Input: part model. Units: mm. Frame: model coordinates. A direction names the side the tool comes from. Coordinates: 2 decimals unless noted, no trailing zeros. Loops run counter-clockwise (first coordinate to the right, second up) from the corner with the lowest first, then second, coordinate; pieces in that order, holes last.
(1) Section C-C, the plane z = -12. Return loops of the section in (x, y).
(2) Section D-D, the plane y = 12. Return loops of the section in (x, z).
(3) Section A-A, the plane z = 0. Return loops of the section in (x, y).
(4) Mould query, pull axis Y, two halves, no side actions, for faces 1 (the face through (-15, -0.762, 1)), 2 (the face through (-20, 20.238, 1)), 3 (the face through (-15.266, 10.836, -49.93)), 4 (the face through (-16, 11, -60)). Classes: released by +Y, released by -Y, zero draft, split by the parting line, or undercut.
(5) Set-up query: faces 5 (the face through (-16, 11, 60)), 6 (the face through (-21, 17.238, 1)). Return all of +Z, -Z, +X, -X, +Y, -Y with unobstructed straight access to the full face (end or side cutting, diameter ignored); none if empty.
(6) Section B-B, the plane z = 50. Return loops of the section in (x, y), then the cut area to 4 significant figures.
(7) Contact query for flat-ended pins moving along their axis: P1, Ø3, axis at y = 9.24, z = -50, coming from the -X side; P2, Ø5, axis at x = -22.78, z = 0, coming from the -Y side. Output: stop coordinate, or through.
(8) Line query: L1, parallel to X at y = 18.05, z = 50; L2, parallel to X at y = 19.4, z = 0; L3, parallel to Y at x = -21.5, z = -43. Output: solid intervals per line, ascending.
```python
from build123d import *

# Parameters (mm, degrees)
EXTRUDE_1_DEPTH     = 60
FILLET_2_R          = 1
FILLET_3_R          = 1
SKETCH_6_R          = 1.6
CUT_EXTRUDE_3_DEPTH = 10
SKETCH_7_R          = 1.6
SKETCH_7_R_2        = 3.879374182
CUT_EXTRUDE_4_DEPTH = 10


with BuildPart() as part:
    # 草图1 → 凸台-拉伸1 (new, symmetric)
    with BuildSketch(Plane.XY):
        Polygon((-13.744850262, -0.762431654), (-13.744850262, 20.237568346), (-24.994850262, 20.237568346), (-24.994850262, 17.237568346), (-16.744850262, 17.237568346), (-16.744850262, -0.762431654), align=None)
    extrude(amount=EXTRUDE_1_DEPTH, both=True)

    # 圆角2
    fillet_2_edges = [part.edges().sort_by_distance(p)[0] for p in [
        (-13.744850262, 20.237568346, 0),
    ]]
    fillet(fillet_2_edges, radius=FILLET_2_R)

    # 圆角3
    fillet_3_edges = [part.edges().sort_by_distance(p)[0] for p in [
        (-16.744850262, 17.237568346, 0),
    ]]
    fillet(fillet_3_edges, radius=FILLET_3_R)

    # 草图6 → 切除-拉伸3 (cut)
    with BuildSketch(Plane.ZY.offset(16.744850262)):
        with Locations(Location((50, 9.237568346, 0), (0, 0, 270))):
            Circle(SKETCH_6_R)
        with Locations(Location((-50, 9.237568346, 0), (0, 0, 270))):
            Circle(SKETCH_6_R)
    extrude(amount=-CUT_EXTRUDE_3_DEPTH, mode=Mode.SUBTRACT)

    # 草图7 → 切除-拉伸4 (cut)
    with BuildSketch(Plane.XZ.offset(-17.237568346)):
        with Locations(Location((-21.994850262, -50, 0), (0, 0, 270))):
            Circle(SKETCH_7_R)
        with Locations(Location((-21.994850262, 50, 0), (0, 0, 270))):
            Circle(SKETCH_7_R)
        with Locations(Location((-22.777733305, 0, 0), (0, 0, 270))):
            Circle(SKETCH_7_R)
        with Locations((-6.137965093, 23.424487804)):
            Circle(SKETCH_7_R_2)
    extrude(amount=-CUT_EXTRUDE_4_DEPTH, mode=Mode.SUBTRACT)


solid = part.part
```
Report:
1. outline: (-24.99, 17.24) - (-17.74, 17.24) arc R1 cw to (-16.74, 16.24) - (-16.74, -0.76) - (-13.74, -0.76) - (-13.74, 19.24) arc R1 ccw to (-14.74, 20.24) - (-24.99, 20.24) - close
2. outline: (-16.74, -60) - (-13.74, -60) - (-13.74, 60) - (-16.74, 60) - close
3. outline: (-24.99, 17.24) - (-24.38, 17.24) - (-24.38, 20.24) - (-24.99, 20.24) - close; (-21.18, 17.24) - (-17.74, 17.24) arc R1 cw to (-16.74, 16.24) - (-16.74, -0.76) - (-13.74, -0.76) - (-13.74, 19.24) arc R1 ccw to (-14.74, 20.24) - (-21.18, 20.24) - close
4. face 1: released by -Y
4. face 2: released by +Y
4. face 3: undercut
4. face 4: zero draft
5. face 5: +Z, +X, -X, +Y, -Y
5. face 6: +Z, -Z, -X, -Y
6. outline: (-24.99, 17.24) - (-23.59, 17.24) - (-23.59, 20.24) - (-24.99, 20.24) - close; (-20.39, 17.24) - (-17.74, 17.24) arc R1 cw to (-16.74, 16.24) - (-16.74, 10.84) - (-13.74, 10.84) - (-13.74, 19.24) arc R1 ccw to (-14.74, 20.24) - (-20.39, 20.24) - close; (-16.74, -0.76) - (-13.74, -0.76) - (-13.74, 7.64) - (-16.74, 7.64) - close
6. area: 68.55 mm2
7. P1: passes through
7. P2: stops at y = 17.24
8. L1: x = -24.99 to -23.59, -20.39 to -13.74
8. L2: x = -24.99 to -24.38, -21.18 to -13.76
8. L3: y = 17.24 to 20.24
